```python
from build123d import *

# Parameters (mm, degrees)
BOSS_EXTRUDE1_START         = -15
BOSS_EXTRUDE1_DEPTH         = 30
BOSS_EXTRUDE1_START_2       = -12.7
BOSS_EXTRUDE1_2_OUTLINE_W   = 6
BOSS_EXTRUDE1_2_OUTLINE_H   = 5.949524979
BOSS_EXTRUDE1_2_DEPTH       = 25.4
BOSS_EXTRUDE1_3_OUTLINE_R   = 15
BOSS_EXTRUDE1_3_OUTLINE_R_2 = 4.55
BOSS_EXTRUDE1_3_DEPTH       = 19.994560744
SKETCH4_W                   = 3.6
SKETCH4_H                   = 22.4
CUT_EXTRUDE1_DEPTH          = 6
BOSS_EXTRUDE2_REACH         = 70.216
BOSS_EXTRUDE2_END_RADIUS    = 119.634966004
SKETCH9_R                   = 6.57997386
SKETCH9_R_2                 = 3.45
SKETCH10_W                  = 5.949524979
SKETCH10_H                  = 2.3
BOSS_EXTRUDE3_DEPTH         = 6


with BuildPart() as part:
    # Boss-Extrude1: read off the stored shape, not the designer's step
    # Boss-Extrude1 outline → Boss-Extrude1 (new body)
    with BuildSketch(Plane(origin=(0, 0, 0), x_dir=(1, 0, 0), z_dir=(0, 1, 0)).offset(BOSS_EXTRUDE1_START)):
        with BuildLine():
            Line((-50, -30), (-50, -35.949524979))
            ThreePointArc((-50, -35.949524979), (-25.592440765, -27.769436157), (0, -25))
            ThreePointArc((0, -25), (25.592440765, -27.769436157), (50, -35.949524979))
            Line((50, -35.949524979), (50, -30))
            ThreePointArc((50, -30), (27.810549479, -22.327809439), (4.550000287, -19.13702996))
            ThreePointArc((4.550000287, -19.13702996), (2.275411741, -19.072115713), (0, -19.050475021))
            ThreePointArc((0, -19.050475021), (-25.592440765, -21.819911178), (-50, -30))
        make_face()
    extrude(amount=BOSS_EXTRUDE1_DEPTH)

    # Boss-Extrude1 2 outline → Boss-Extrude1 2 (add)
    with BuildSketch(Plane(origin=(0, 0, 0), x_dir=(1, 0, 0), z_dir=(0, 1, 0)).offset(BOSS_EXTRUDE1_START_2)):
        with Locations((-53, -32.97476249)):
            Rectangle(BOSS_EXTRUDE1_2_OUTLINE_W, BOSS_EXTRUDE1_2_OUTLINE_H)
    extrude(amount=BOSS_EXTRUDE1_2_DEPTH)

    # Boss-Extrude1 3 outline → Boss-Extrude1 3 (add)
    with BuildSketch(Plane.XY):
        Circle(BOSS_EXTRUDE1_3_OUTLINE_R)
        Circle(BOSS_EXTRUDE1_3_OUTLINE_R_2, mode=Mode.SUBTRACT)
    extrude(amount=BOSS_EXTRUDE1_3_DEPTH)

    # Sketch4 → Cut-Extrude1 (cut)
    with BuildSketch(Plane.XY.offset(35.949524979)):
        with Locations((-53, 0)):
            Rectangle(SKETCH4_W, SKETCH4_H)
    extrude(amount=-CUT_EXTRUDE1_DEPTH, mode=Mode.SUBTRACT)

    # Sketch8 → CBORE for M8 Hex Head Bolt1 (revolve, cut)
    with BuildSketch(Plane.YZ.offset(40.380081118)):
        Polygon((0, 0), (0, 35.949524979), (4.5, 35.949524979), (4.5, 5.68), (9.005, 5.68), (9.005, 0.025), (9.03, 0), align=None)
    revolve(axis=Axis((40.380081118, 0, -6.35), (0, 0, 1)), mode=Mode.SUBTRACT)

    # Boss-Extrude2: up to this cylinder (the profile starts outside it)
    boss_extrude2_end = Plane(origin=(0, 0, 138.685441025), z_dir=(0, -1, 0)) * Cylinder(BOSS_EXTRUDE2_END_RADIUS, 380.701932008, mode=Mode.PRIVATE)
    # Sketch9 → Boss-Extrude2 (add, up to the surface)
    with BuildSketch(Plane(origin=(0, 0, 0), x_dir=(-1, 0, 0), z_dir=(0, 0, -1)), mode=Mode.PRIVATE) as boss_extrude2_sk1:
        Circle(SKETCH9_R)
        Circle(SKETCH9_R_2, mode=Mode.SUBTRACT)
    boss_extrude2_tool1 = extrude(boss_extrude2_sk1.sketch, amount=-BOSS_EXTRUDE2_REACH, mode=Mode.PRIVATE) - boss_extrude2_end
    add(boss_extrude2_tool1.solids().sort_by_distance((6.393864, 0, 0))[0])

    # Sketch10 → Boss-Extrude3 (add)
    with BuildSketch(Plane.ZY.offset(50)):
        with Locations((32.97476249, 13.85)):
            Rectangle(SKETCH10_W, SKETCH10_H)
        with Locations((32.97476249, -13.85)):
            Rectangle(SKETCH10_W, SKETCH10_H)
    extrude(amount=BOSS_EXTRUDE3_DEPTH)


solid = part.part
```
Here's how the part is built. I have some questions about the finished solid (model axes, mm). A direction names the side the tool comes from. Round coordinates to 2 decimals unless told otherwise and drop trailing zeros. Order: outer loops, then holes, each group sorted by start corner. A loop starts at its lowest first (then second) coordinate and runs counter-clockwise, first axis right, second up. Notation, with made-up numbers: M 60,-1.5 L 74,-1.5 A28 cw 74,18.5 Z; hole C 78,-5.75 d8. An arc over 180 degrees is marked long. Use CSV: the item, a comma, the result in double quotes.
1) I want a section at C-C (y = -7). List the corners of the cut face in (x, z) for me, then the cut area to 3 significant figures.
Taken from the geometry:
outline,"M -56,30 L -54.8,30 L -54.8,35.95 L -56,35.95 Z; M -51.2,30 L -50,30 A119.63 ccw -13.27,19.79 L -13.27,0 L 13.27,0 L 13.27,19.79 A119.63 ccw 50,30 L 50,35.95 A119.63 cw -50,35.95 L -51.2,35.95 Z"
area,"1,120 mm^2"
2) On a 3-axis mill with a long thin cutter (end or side, diameter ignored), from which of +Z, -Z, +X, -X, +Y, -Y can I reach the whole of each face in a straight line? I mean faces 4 (the flat face through (-54.8, 0, 33)), 5 (the flat face through (50, 0, 33)), 6 (the cylindrical face through (0.45, 3.42, 9.42)). Say none if no direction works.
Taken from the geometry:
face 4,"+Z, -Z"
face 5,"+Z, -Z, +X, +Y, -Y"
face 6,"-Z"
3) I want a section at D-D (z = 12.5). List the corners of the cut face in (x, y) for me, then the cut area to 3 significant figures.
Taken from the geometry:
outline,"C 0,0 d30; hole C 0,0 d6.9"
area,"669 mm^2"
4) I need wall thicknesses on line 1 along X through (y, z) = (0, 4); line 2 along Z through (x, y) = (1, 8). Which ranges of each line are inside material? Lowest first, please. Write a range as [from, to].
Taken from the geometry:
line 1,"[-15, -3.45], [3.45, 15]"
line 2,"[0, 25]"
5) I'm going to push flat-ended pins straight in: P1, Ø3, axis at x = -15, y = 1.5, coming from the +Z side; P2, Ø10.5, axis at x = 40.38, y = 0, coming from the -Z side; P3, Ø2, axis at y = -2.5, z = 8, coming from the -X side. Where does each tip first touch, or does it pass through?
Taken from the geometry:
P1,"z = 26.14"
P2,"z = 24.32"
P3,"x = -14.92"
6) I want a section at B-B (y = 2). List the corners of the cut face in (x, z) for me.
Taken from the geometry:
outline,"M -56,30 L -54.8,30 L -54.8,35.95 L -56,35.95 Z; M -51.2,30 L -50,30 A119.63 ccw -14.87,19.98 L -14.87,0 L -2.81,0 L -2.81,19.08 A119.63 ccw 2.81,19.08 L 2.81,0 L 14.87,0 L 14.87,19.98 A119.63 ccw 36.35,24.71 L 36.35,30.66 A119.63 cw -50,35.95 L -51.2,35.95 Z; M 44.41,27.6 A119.63 ccw 50,30 L 50,35.95 A119.63 cw 44.41,33.55 Z"
7) If we mould it in two halves opening along Y, with no side actions, what happens to faces 1 (the cylindrical face through (-14.985, 0.66, 9.857)), 2 (the flat face through (-51, 0, 30)), 3 (the flat face through (-51.2, 0, 33))? For each: pulls with the +Y half, pulls with the -Y half, needs draft (parallel to the pull), parting line crosses it, or undercut.
Taken from the geometry:
face 1,"parting line crosses it"
face 2,"needs draft"
face 3,"undercut"
8) I want a section at A-A (z = 29). List the corners of the cut face in (x, y) for me.
Taken from the geometry:
outline,"M -47.77,-15 L -30.68,-15 L -30.68,15 L -47.77,15 Z; M 30.68,-15 L 47.77,-15 L 47.77,15 L 30.68,15 Z; hole C 40.38,0 d9"
